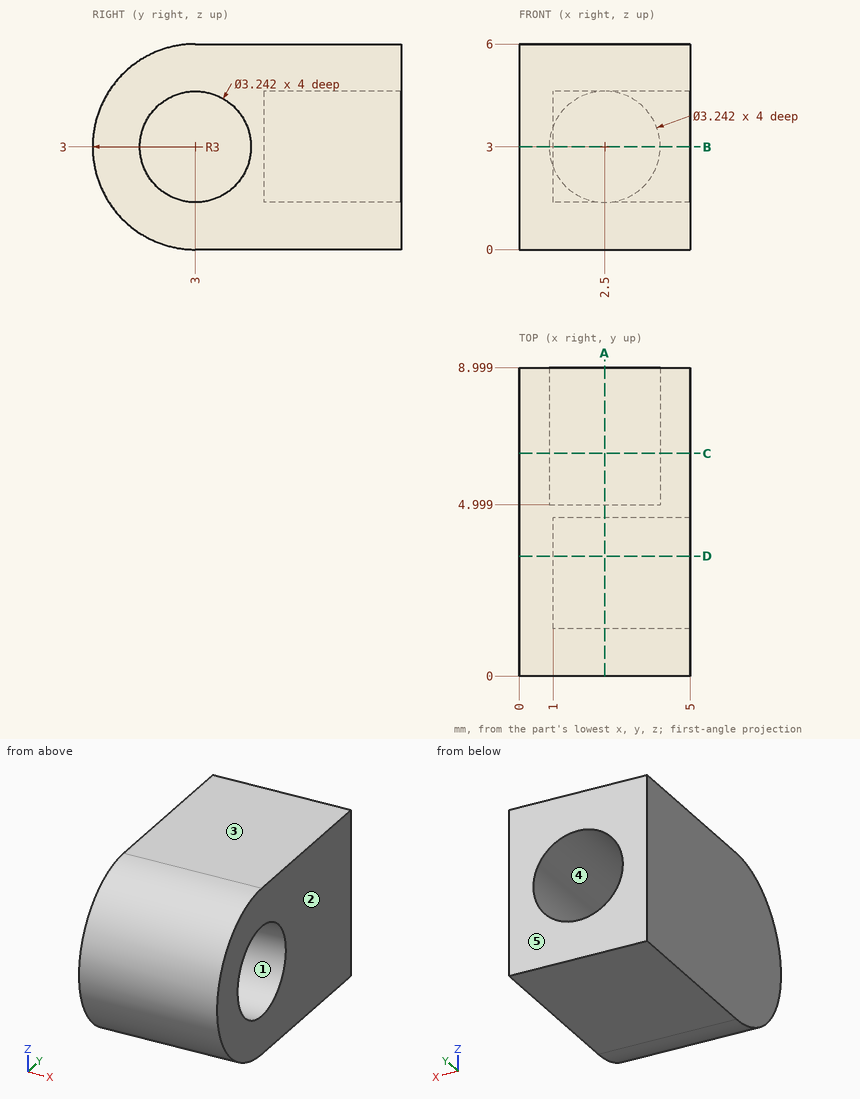
Study the drawing (mm; zero at the part's minimum x, y, z) and answer. A direction names the side the tool comes from. Coordinates: 2 decimals unless noted, no trailing zeros. Write each loop counter-clockwise with the first axis right and the second up, starting at its lowest first coordinate (ties: lowest second). Pieces come first, ordered by that corner, then holes.
Q1. Section B-B, the plane z = 3 is taken. Write down the section's boundary in (x, y).
Returned:
outline: (0, 0) - (5, 0) - (5, 1.38) - (1, 1.38) - (1, 4.62) - (5, 4.62) - (5, 9) - (4.12, 9) - (4.12, 5) - (0.88, 5) - (0.88, 9) - (0, 9) - close
Q2. Section C-C, the plane y = 6.5 is taken. Write down the section's boundary in (x, z).
Returned:
outline: (0, 0) - (5, 0) - (5, 6) - (0, 6) - close; hole circle Ø3.24 at (2.5, 3)
Q3. Find the intervals of material crossed by line 1 along X through (y, z) = (6.9, 3); line 2 along Y through (x, z) = (2.75, 3); line 3 along Z through (x, y) = (2.5, 7.15), in increasing order.
Returned:
line 1: x = 0 to 0.88, 4.12 to 5
line 2: y = 0 to 1.38, 4.62 to 5
line 3: z = 0 to 1.38, 4.62 to 6
Q4. Section D-D, the plane y = 3.5 is taken. Write down the section's boundary in (x, z).
Returned:
outline: (0, 0) - (5, 0) - (5, 1.46) - (1, 1.46) - (1, 4.54) - (5, 4.54) - (5, 6) - (0, 6) - close
Q5. Given P1, Ø1, axis at y = 3.5, z = 3.5, coming from the +X side; P2, Ø1, axis at x = 2.5, z = 3.5, coming from the +Y side; P3, Ø1.5, axis at x = 2, z = 2, coming from the -Y side, each flat-ended and moving along its own axis, determine where each tip first touches the part or whether it passes through.
Returned:
P1: stops at x = 1
P2: stops at y = 5
P3: stops at y = 0.01
Q6. The mould has two halves that part along Z. Classify the marked faces 1, 2 and 3: released by +Z, released by -Z, zero draft, split by the parting line, or undercut.
Returned:
face 1: undercut
face 2: zero draft
face 3: released by +Z
Q7. Section A-A, the plane x = 2.5 is taken. Write down the section's boundary in (y, z).
Returned:
outline: (3, 0) - (9, 0) - (9, 1.38) - (5, 1.38) - (5, 4.62) - (9, 4.62) - (9, 6) - (3, 6) arc R3 ccw to start; hole circle Ø3.24 at (3, 3)
Q8. Which of the six approach directions +Z, -Z, +X, -X, +Y, -Y give full straight-line access (tool end or side, diameter ignored) to the marked faces 4 and 5?
Returned:
face 4: +Y
face 5: +Z, -Z, +X, -X, +Y
